Input: part model. Units: mm. Frame: model coordinates. A direction names the side the tool comes from. Coordinates: 2 decimals unless noted, no trailing zeros. Write each loop counter-clockwise with the first axis right and the second up, starting at its lowest first coordinate (ties: lowest second). Pieces come first, ordered by that corner, then holes. Notation, with made-up numbers: (20.25, 49.25) - (61.25, 49.25) arc R23 ccw to (61.25, 64.25) - close; hole circle Ø6 at (32, 38). An arc over 180 degrees is marked (long way). One line per question, with ' | ' between items. Start each with the question number.
1) First-contact query: P1, Ø8, axis at y = -23, z = 12.5, coming from the +X side; P2, Ø6, axis at x = 2.5, y = 0.5, coming from the -Z side; P3, Ø3, axis at x = 19.5, z = 0.5, coming from the -Y side; P4, Ø12, axis at x = 0.5, z = 1, coming from the +Y side. Flat tips, straight axial feed; report the tip coordinate or a pass-through.
2) Section query C-C on y = -11. Return loops of the section in (x, z).
3) Reachability of faces 1 (the flat face through (-16, -27, 9)), 2 (the flat face through (-10, 32, -7)), 3 (the flat face through (-17.768, 25.535, -3.133)), 4 (the cylindrical face through (14.195, -25.605, 7.383)), 5 (the flat face through (-17.768, 25.535, 3.133)) from +Z, -Z, +X, -X, +Y, -Y: full face, straight path, thin tool, end or side. Return the list, or none.
4) Section query B-B on z = 0. Return loops of the section in (x, y).
5) Draft query along Z for faces 6 (the flat face through (17.69, 25.54, -3.12)), 7 (the cylindrical face through (21, 26, 0)), 8 (the flat face through (-12, -25, 12)), 9 (the flat face through (-12, -18, -2)). Return one class per face: released by +Z, released by -Z, zero draft, split by the parting line, or undercut.
6) Line query: line 1 (X direction, y = -2, z = 0); line 2 (Z direction, x = -0.5, y = 21.5); line 3 (Z direction, x = -9, y = -6.5). Output: solid intervals per line, ascending.
7) Section query A-A on x = 0. Return loops of the section in (y, z), and give its area (3 significant figures).
8) Section query D-D on z = -8. Give the number of separate pieces and of enclosed holes in the cut face, and give its area (3 significant figures).
```python
from build123d import *

# Parameters (mm, degrees)
SKETCH2_W          = 6
SKETCH2_H          = 5
REVOLVE2_ANGLE     = 20
SKETCH3_W          = 3
SKETCH3_H          = 10
SKETCH3_H_2        = 11
CUT_REVOLVE1_ANGLE = 25
SKETCH4_W          = 3
SKETCH4_H          = 5
SKETCH4_H_2        = 4
CUT_REVOLVE2_ANGLE = 45


with BuildPart() as part:
    # Sketch1 → Revolve1 (revolve)
    with BuildSketch(Plane.XY, mode=Mode.PRIVATE) as revolve1_sk:
        Polygon((12, 32), (12, -18), (16, -18), (16, -33), (19, -33), (19, -18), (15, -8), (15, 32), align=None)
    revolve(revolve1_sk.sketch.rotate(Axis((0, 40.467735012, 0), (0, -1, 0)), 90), axis=Axis((0, 40.467735012, 0), (0, -1, 0)))

    # Sketch2 → Revolve2 (revolve, symmetric)
    with BuildSketch(Plane.XY) as revolve2_sk:
        with Locations((18, 25.5)):
            Rectangle(SKETCH2_W, SKETCH2_H)
        with Locations((-18, 25.5)):
            Rectangle(SKETCH2_W, SKETCH2_H)
    revolve(axis=Axis((0, 45.306661743, 0), (0, -1, 0)), revolution_arc=REVOLVE2_ANGLE / 2)
    revolve(revolve2_sk.sketch, axis=Axis((0, 45.306661743, 0), (0, 1, 0)), revolution_arc=REVOLVE2_ANGLE / 2)

    # Sketch3 → Cut-Revolve1 (revolve, symmetric, cut)
    with BuildSketch(Plane.XY) as cut_revolve1_sk:
        with Locations((-17.5, -28)):
            Rectangle(SKETCH3_W, SKETCH3_H)
        with Locations((17.5, -27.5)):
            Rectangle(SKETCH3_W, SKETCH3_H_2)
    revolve(axis=Axis((0, -11.020729768, 0), (0, -1, 0)), revolution_arc=CUT_REVOLVE1_ANGLE / 2, mode=Mode.SUBTRACT)
    revolve(cut_revolve1_sk.sketch, axis=Axis((0, -11.020729768, 0), (0, 1, 0)), revolution_arc=CUT_REVOLVE1_ANGLE / 2, mode=Mode.SUBTRACT)

    # Sketch4 → Cut-Revolve2 (revolve, cut)
    with BuildSketch(Plane.XY):
        with Locations((17.5, -24.5)):
            Rectangle(SKETCH4_W, SKETCH4_H)
        with Locations((-17.5, -25)):
            Rectangle(SKETCH4_W, SKETCH4_H_2)
    revolve(axis=Axis((0, -42.004114959, 0), (0, 1, 0)), revolution_arc=CUT_REVOLVE2_ANGLE, mode=Mode.SUBTRACT)


solid = part.part
```
Answer key:
1) P1: x = 16.99 | P2: z = -15 | P3: y = -22 | P4: through
2) outline: circle Ø32.4 at (0, 0); hole circle Ø24 at (0, 0)
3) face 1: -X | face 2: +Z, -Z, +X, -X, +Y | face 3: -Z, +Y | face 4: -Y | face 5: +Z, +Y
4) outline: (-21, 23) - (-15, 23) - (-15, -8) - (-19, -18) - (-19, -23) - (-16, -23) - (-16, -18) - (-12, -18) - (-12, 32) - (-15, 32) - (-15, 28) - (-21, 28) - close; (12, -18) - (16, -18) - (16, -22) - (19, -22) - (19, -18) - (15, -8) - (15, 23) - (21, 23) - (21, 28) - (15, 28) - (15, 32) - (12, 32) - close
5) face 6: released by -Z | face 7: split by the parting line | face 8: undercut | face 9: undercut
6) line 1: -15 to -12, 12 to 15 | line 2: -14.99 to -11.99, 11.99 to 14.99 | line 3: -12 to -7.94, 7.94 to 12
7) outline: (-33, -19) - (-18, -19) - (-8, -15) - (32, -15) - (32, -12) - (-18, -12) - (-18, -16) - (-33, -16) - close; (-33, 16) - (-18, 16) - (-18, 12) - (32, 12) - (32, 15) - (-8, 15) - (-18, 19) - (-33, 19) - close | area: 430 mm²
8) separate pieces: 3 | enclosed holes: 0 | area: 505 mm²
